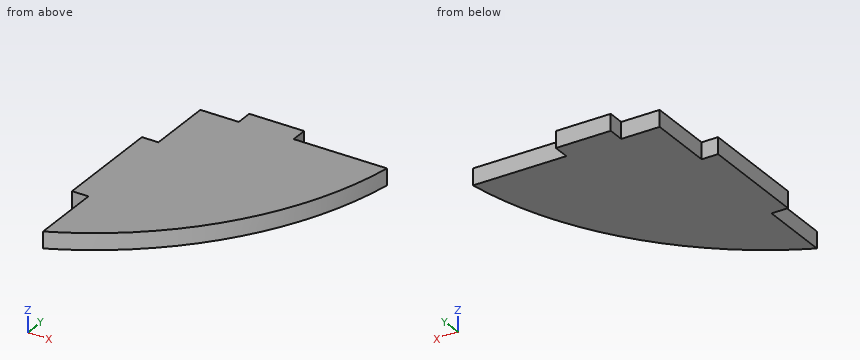
from build123d import *

# Parameters (mm, degrees)
EXTRUDE_1_DEPTH = 1.5


with BuildPart() as part:
    # 草图2 → 凸台-拉伸1 (new body, symmetric)
    with BuildSketch(Plane.XY):
        with BuildLine():
            Line((0, 45), (0, 33))
            Line((0, 33), (-3, 33))
            Line((-3, 33), (-3, 13))
            Line((-3, 13), (0, 13))
            Line((0, 13), (0, 0))
            ThreePointArc((0, 0), (22.61707334, 18.255989032), (34, 45))
            Line((34, 45), (17, 45))
            Line((17, 45), (17, 48))
            Line((17, 48), (7, 48))
            Line((7, 48), (7, 45))
            Line((7, 45), (0, 45))
        make_face()
    extrude(amount=EXTRUDE_1_DEPTH, both=True)


solid = part.part
Could you check a few things on this model? Use its own coordinates, in mm. Give positions to 0.01 mm unless a question says otherwise; leave off trailing zeros. Order: outer loops, then holes, each group sorted by start corner. A loop starts at its lowest first (then second) coordinate and runs counter-clockwise, first axis right, second up. Notation, with made-up numbers: (72.25, 66) - (90.25, 66) arc R9 cw to (90.25, 81) - close; hole circle Ø1 at (38, 0.5). An arc over 180 degrees is marked (long way). Return JSON: item names as keys, results as strings. Group by question number.
Q1. Will these pins go through, and if not, where does the flat tip stop? pin 1 Ø0.9 at (y, z) = (46, -0.5) entering from +X; pin 2 Ø1.5 at (x, z) = (26, 0.5) entering from +Y; pin 3 Ø1.5 at (y, z) = (11.5, -0.5) entering from -X.
Q2. Suppose I cut it at C-C, the plane y = 18.5. Please give me the cut outline in (x, z), and give its area (3 significant figures).
Q3. Please list where these lines run through material, in increasing order: line 1 along Y through (x, z) = (0.5, 1.1); line 2 along X through (y, z) = (15, -0.3); line 3 along X through (y, z) = (35.5, -0.4). Write a range as [from, to].
Q4. Suppose I cut it at A-A, the plane z = 0.7. Please give me the cut outline in (x, y), and give its area (3 significant figures).
Q5. Suppose I cut it at B-B, the plane x = 9. Please give me the cut outline in (y, z).
Resolved:
{
 "1": {"pin 1": "stops at x = 17", "pin 2": "stops at y = 45", "pin 3": "stops at x = 0"},
 "2": {"outline": "(-3, -1.5) - (22.8, -1.5) - (22.8, 1.5) - (-3, 1.5) - close", "area": "77.4 mm2"},
 "3": {"line 1": "y = [0.23, 45]", "line 2": "x = [-3, 19.97]", "line 3": "x = [0, 31.68]"},
 "4": {"outline": "(-3, 13) - (0, 13) - (0, 0) arc R60 ccw to (34, 45) - (17, 45) - (17, 48) - (7, 48) - (7, 45) - (0, 45) - (0, 33) - (-3, 33) - close", "area": "1,120 mm2"},
 "5": {"outline": "(5.17, -1.5) - (48, -1.5) - (48, 1.5) - (5.17, 1.5) - close"}
}
